Design review of the part built by this model. Coordinates are the model's own, in mm. Face numbers are marked on the shaded views. A direction names the side the tool comes from. Give positions to 0.01 mm unless a question says otherwise; leave off trailing zeros. Order: outer loops, then holes, each group sorted by start corner. A loop starts at its lowest first (then second) coordinate and runs counter-clockwise, first axis right, second up. Notation, with made-up numbers: (35, 4.25) -> (49, 4.25) arc R25 cw to (49, 37.25) -> close; hole circle Ø4 at (71.25, 22.5). An arc over 180 degrees is marked (long way). Use a Markdown table: item, result. Add a question column.
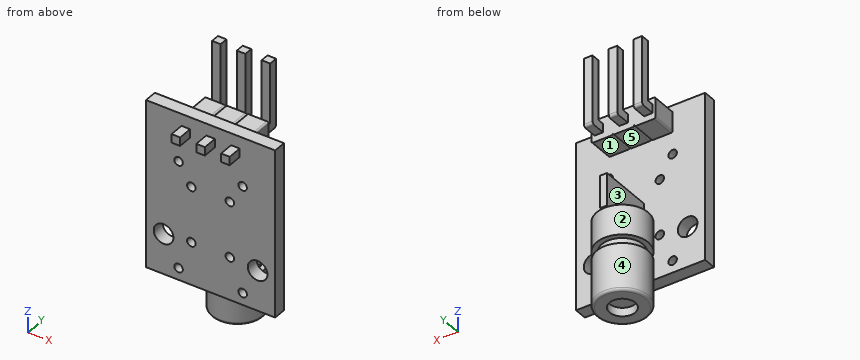
```python
from build123d import *

# Parameters (mm, degrees)
SKETCH1_W           = 15.1
SKETCH1_H           = 19.6
BOSS_EXTRUDE1_DEPTH = 1.5
SKETCH2_W           = 1
SKETCH2_H           = 1
BOSS_EXTRUDE2_DEPTH = 1.7
BOSS_EXTRUDE3_DEPTH = 2.9
SKETCH4_W           = 1
SKETCH4_H           = 1
BOSS_EXTRUDE4_DEPTH = 1.8
SKETCH5_W           = 1
SKETCH5_H           = 1
BOSS_EXTRUDE5_DEPTH = 7
SKETCH7_W           = 0.8
SKETCH7_H           = 3.8
BOSS_EXTRUDE6_DEPTH = 6.3
SKETCH8_R           = 3
BOSS_EXTRUDE7_DEPTH = 3.5
SKETCH9_R           = 2.4
BOSS_EXTRUDE8_DEPTH = 1
SKETCH10_R          = 3
BOSS_EXTRUDE9_DEPTH = 5.5
FILLET1_R           = 0.3
SKETCH11_R          = 1.5
CUT_EXTRUDE1_DEPTH  = 1
SKETCH12_R          = 1.15
CUT_EXTRUDE2_DEPTH  = 19.271631016
CUT_EXTRUDE3_REACH  = 20.842
SKETCH13_R          = 0.5
CUT_EXTRUDE4_REACH  = 20.842
SKETCH14_R          = 0.5
FILLET2_R           = 0.2
FILLET3_R           = 0.05
FILLET5_R           = 0.3


with BuildPart() as part:
    # Sketch1 → Boss-Extrude1 (new body)
    with BuildSketch(Plane(origin=(0, 0, 0), x_dir=(1, 0, 0), z_dir=(0, 1, 0))):
        Rectangle(SKETCH1_W, SKETCH1_H)
    extrude(amount=BOSS_EXTRUDE1_DEPTH)

    # Sketch2 → Boss-Extrude2 (add)
    with BuildSketch(Plane.XZ):
        with Locations((0, 7.9)):
            Rectangle(SKETCH2_W, SKETCH2_H)
        with Locations((2.9, 7.9)):
            Rectangle(SKETCH2_W, SKETCH2_H)
        with Locations((-2.9, 7.9)):
            Rectangle(SKETCH2_W, SKETCH2_H)
    extrude(amount=BOSS_EXTRUDE2_DEPTH)

    # Sketch3 → Boss-Extrude3 (add)
    with BuildSketch(Plane(origin=(0, 1.5, 0), x_dir=(1, 0, 0), z_dir=(0, 1, 0))):
        with BuildLine():
            Line((-3.75, -9.15), (-3.75, -6.65))
            Line((-3.75, -6.65), (-1.45, -6.65))
            ThreePointArc((-1.45, -6.65), (-1.308578644, -6.708578644), (-1.25, -6.85))
            ThreePointArc((-1.25, -6.85), (-1.191421356, -6.708578644), (-1.05, -6.65))
            Line((-1.05, -6.65), (1.05, -6.65))
            ThreePointArc((1.05, -6.65), (1.191421356, -6.708578644), (1.25, -6.85))
            ThreePointArc((1.25, -6.85), (1.308578644, -6.708578644), (1.45, -6.65))
            Line((1.45, -6.65), (3.75, -6.65))
            Line((3.75, -6.65), (3.75, -9.15))
            Line((3.75, -9.15), (1.45, -9.15))
            ThreePointArc((1.45, -9.15), (1.308578644, -9.091421356), (1.25, -8.95))
            ThreePointArc((1.25, -8.95), (1.191421356, -9.091421356), (1.05, -9.15))
            Line((1.05, -9.15), (-1.05, -9.15))
            ThreePointArc((-1.05, -9.15), (-1.191421356, -9.091421356), (-1.25, -8.95))
            ThreePointArc((-1.25, -8.95), (-1.308578644, -9.091421356), (-1.45, -9.15))
            Line((-1.45, -9.15), (-3.75, -9.15))
        make_face()
    extrude(amount=BOSS_EXTRUDE3_DEPTH)

    # Sketch4 → Boss-Extrude4 (add)
    with BuildSketch(Plane(origin=(0, 4.4, 0), x_dir=(1, 0, 0), z_dir=(0, 1, 0))):
        with Locations((-2.9, -7.9)):
            Rectangle(SKETCH4_W, SKETCH4_H)
        with Locations((0, -7.9)):
            Rectangle(SKETCH4_W, SKETCH4_H)
        with Locations((2.9, -7.9)):
            Rectangle(SKETCH4_W, SKETCH4_H)
    extrude(amount=BOSS_EXTRUDE4_DEPTH)

    # Sketch5 → Boss-Extrude5 (add)
    with BuildSketch(Plane.XY.offset(8.4)):
        with Locations((-2.9, 5.7)):
            Rectangle(SKETCH5_W, SKETCH5_H)
        with Locations((0, 5.7)):
            Rectangle(SKETCH5_W, SKETCH5_H)
        with Locations((2.9, 5.7)):
            Rectangle(SKETCH5_W, SKETCH5_H)
    extrude(amount=BOSS_EXTRUDE5_DEPTH)

    # Sketch7 → Boss-Extrude6 (add)
    with BuildSketch(Plane(origin=(0, 1.5, 0), x_dir=(1, 0, 0), z_dir=(0, 1, 0))):
        with Locations((0, 2.3)):
            Rectangle(SKETCH7_W, SKETCH7_H)
    extrude(amount=BOSS_EXTRUDE6_DEPTH)

    # Sketch8 → Boss-Extrude7 (add)
    with BuildSketch(Plane(origin=(0, 0, -4.2), x_dir=(-1, 0, 0), z_dir=(0, 0, -1))):
        with Locations(Location((0, 4.6, 0), (0, 0, 262.337744339))):
            Circle(SKETCH8_R)
    extrude(amount=BOSS_EXTRUDE7_DEPTH)

    # Sketch9 → Boss-Extrude8 (add)
    with BuildSketch(Plane(origin=(0, 0, -7.7), x_dir=(-1, 0, 0), z_dir=(0, 0, -1))):
        with Locations((0, 4.6)):
            Circle(SKETCH9_R)
    extrude(amount=BOSS_EXTRUDE8_DEPTH)

    # Sketch10 → Boss-Extrude9 (add)
    with BuildSketch(Plane(origin=(0, 0, -8.7), x_dir=(-1, 0, 0), z_dir=(0, 0, -1))):
        with Locations(Location((0, 4.6, 0), (0, 0, 262.337744339))):
            Circle(SKETCH10_R)
    extrude(amount=BOSS_EXTRUDE9_DEPTH)

    # Fillet1
    fillet1_edges = [part.edges().sort_by_distance(p)[0] for p in [
        (-0.4, 7.573213749, -14.2),
    ]]
    fillet(fillet1_edges, radius=FILLET1_R)

    # Sketch11 → Cut-Extrude1 (cut)
    with BuildSketch(Plane(origin=(0, 0, -14.2), x_dir=(-1, 0, 0), z_dir=(0, 0, -1))):
        with Locations((0, 4.6)):
            Circle(SKETCH11_R)
    extrude(amount=-CUT_EXTRUDE1_DEPTH, mode=Mode.SUBTRACT)

    # Sketch12 → Cut-Extrude2 (cut, through all)
    with BuildSketch(Plane(origin=(0, 1.5, 0), x_dir=(1, 0, 0), z_dir=(0, 1, 0))):
        with Locations(Location((-5.5, 5.1, 0), (0, 0, 270))):
            Circle(SKETCH12_R)
        with Locations(Location((5.5, 5.1, 0), (0, 0, 270))):
            Circle(SKETCH12_R)
    extrude(amount=-CUT_EXTRUDE2_DEPTH, mode=Mode.SUBTRACT)

    # Sketch13 → Cut-Extrude3 (cut, up to next)
    with BuildSketch(Plane.XZ, mode=Mode.PRIVATE) as cut_extrude3_sk1:
        with Locations(Location((-2.25, -4.8, 0), (0, 0, 270))):
            Circle(SKETCH13_R)
    cut_extrude3_tool1 = extrude(cut_extrude3_sk1.sketch, amount=-CUT_EXTRUDE3_REACH, mode=Mode.PRIVATE) & part.part
    # Sketch13 → Cut-Extrude3 (cut, up to next)
    with BuildSketch(Plane.XZ, mode=Mode.PRIVATE) as cut_extrude3_sk2:
        with Locations(Location((2.25, -4.8, 0), (0, 0, 270))):
            Circle(SKETCH13_R)
    cut_extrude3_tool2 = extrude(cut_extrude3_sk2.sketch, amount=-CUT_EXTRUDE3_REACH, mode=Mode.PRIVATE) & part.part
    # Sketch13 → Cut-Extrude3 (cut, up to next)
    with BuildSketch(Plane.XZ, mode=Mode.PRIVATE) as cut_extrude3_sk3:
        with Locations(Location((2.25, 1.7, 0), (0, 0, 270))):
            Circle(SKETCH13_R)
    cut_extrude3_tool3 = extrude(cut_extrude3_sk3.sketch, amount=-CUT_EXTRUDE3_REACH, mode=Mode.PRIVATE) & part.part
    # Sketch13 → Cut-Extrude3 (cut, up to next)
    with BuildSketch(Plane.XZ, mode=Mode.PRIVATE) as cut_extrude3_sk4:
        with Locations(Location((-2.25, 1.7, 0), (0, 0, 270))):
            Circle(SKETCH13_R)
    cut_extrude3_tool4 = extrude(cut_extrude3_sk4.sketch, amount=-CUT_EXTRUDE3_REACH, mode=Mode.PRIVATE) & part.part
    add(cut_extrude3_tool1.solids().sort_by_distance((-2.25, 0, -4.8))[0], mode=Mode.SUBTRACT)
    add(cut_extrude3_tool2.solids().sort_by_distance((2.25, 0, -4.8))[0], mode=Mode.SUBTRACT)
    add(cut_extrude3_tool3.solids().sort_by_distance((2.25, 0, 1.7))[0], mode=Mode.SUBTRACT)
    add(cut_extrude3_tool4.solids().sort_by_distance((-2.25, 0, 1.7))[0], mode=Mode.SUBTRACT)

    # Sketch14 → Cut-Extrude4 (cut, up to next)
    with BuildSketch(Plane.XZ, mode=Mode.PRIVATE) as cut_extrude4_sk1:
        with Locations(Location((3.75, 4.1, 0), (0, 0, 270))):
            Circle(SKETCH14_R)
    cut_extrude4_tool1 = extrude(cut_extrude4_sk1.sketch, amount=-CUT_EXTRUDE4_REACH, mode=Mode.PRIVATE) & part.part
    # Sketch14 → Cut-Extrude4 (cut, up to next)
    with BuildSketch(Plane.XZ, mode=Mode.PRIVATE) as cut_extrude4_sk2:
        with Locations(Location((-3.75, 4.1, 0), (0, 0, 270))):
            Circle(SKETCH14_R)
    cut_extrude4_tool2 = extrude(cut_extrude4_sk2.sketch, amount=-CUT_EXTRUDE4_REACH, mode=Mode.PRIVATE) & part.part
    # Sketch14 → Cut-Extrude4 (cut, up to next)
    with BuildSketch(Plane.XZ, mode=Mode.PRIVATE) as cut_extrude4_sk3:
        with Locations(Location((-3.75, -8.4, 0), (0, 0, 270))):
            Circle(SKETCH14_R)
    cut_extrude4_tool3 = extrude(cut_extrude4_sk3.sketch, amount=-CUT_EXTRUDE4_REACH, mode=Mode.PRIVATE) & part.part
    # Sketch14 → Cut-Extrude4 (cut, up to next)
    with BuildSketch(Plane.XZ, mode=Mode.PRIVATE) as cut_extrude4_sk4:
        with Locations(Location((3.75, -8.4, 0), (0, 0, 270))):
            Circle(SKETCH14_R)
    cut_extrude4_tool4 = extrude(cut_extrude4_sk4.sketch, amount=-CUT_EXTRUDE4_REACH, mode=Mode.PRIVATE) & part.part
    add(cut_extrude4_tool1.solids().sort_by_distance((3.75, 0, 4.1))[0], mode=Mode.SUBTRACT)
    add(cut_extrude4_tool2.solids().sort_by_distance((-3.75, 0, 4.1))[0], mode=Mode.SUBTRACT)
    add(cut_extrude4_tool3.solids().sort_by_distance((-3.75, 0, -8.4))[0], mode=Mode.SUBTRACT)
    add(cut_extrude4_tool4.solids().sort_by_distance((3.75, 0, -8.4))[0], mode=Mode.SUBTRACT)

    # Fillet2
    fillet2_edges = [part.edges().sort_by_distance(p)[0] for p in [
        (-3.75, 2.95, 9.15),
        (3.75, 2.95, 9.15),
        (3.75, 2.95, 6.65),
        (-3.75, 2.95, 6.65),
    ]]
    fillet(fillet2_edges, radius=FILLET2_R)

    # Fillet3
    fillet3_edges = [part.edges().sort_by_distance(p)[0] for p in [
        (-2.9, 5.2, 8.4),
        (0, 5.2, 8.4),
        (2.9, 5.2, 8.4),
    ]]
    fillet(fillet3_edges, radius=FILLET3_R)

    # Fillet5
    fillet5_edges = [part.edges().sort_by_distance(p)[0] for p in [
        (-2.9, 6.2, 7.4),
        (0, 6.2, 7.4),
        (2.9, 6.2, 7.4),
    ]]
    fillet(fillet5_edges, radius=FILLET5_R)


solid = part.part
```
1) Add section B-B (z = 4.1). Give the boundary of the cut face in (x, y).
2) Add section D-D (z = -4.8). Give the boundary of the cut face in (x, y).
3) The part is to be moulded in two halves that separate along Z. For the marked faces 4 and 5, say which applies: +Z half, -Z half, draft (parallel to the pull), parting line (faces both ways), or undercut.
4) Machinability: for the marked faces 1, 2 and 3, which of the approach directions +Z, -Z, +X, -X, +Y, -Y give a long, thin tool a straight path to every point of the face, cutting with its end or side? Answer none if there is none.
5) Add section A-A (y = 1). Give the number of separate pieces and of enclosed holes in the cut face, then the cut area to 3 significant figures.
6) Insertion check: pin 1 (1 mm diameter, centred on x = 2, y = 2.5, fed in from +Z); pin 2 (4 mm diameter, centred on y = 7, z = -4, fed in from -X); pin 3 (0.5 mm diameter, centred on y = 5.5, z = 10.5, fed in from +X); pin 4 (5 mm diameter, centred on y = 2.5, z = -9.5, fed in from +X). Each pin has a flat end and moves straight along its axis. Give the tip position at first contact, or say it passes through.
7) For L1, parallel to Y at x = 0, z = -13.35; L2, parallel to X at y = 0.5, z = -5.75; L3, parallel to Z at x = 0.25, y = 5, list the stretches that pass through material, from the lowest coordinate up. Write a range as [from, to].
8) Add section C-C (y = -1). Give the boundary of the cut face in (x, z), then the cut area to 3 significant figures.
Worked answers:
| question | item | result |
|---|---|---|
| 1 | outline | (-7.55, 0) -> (-4.25, 0) -> (-4.25, 1.5) -> (-7.55, 1.5) -> close; (-3.25, 0) -> (3.25, 0) -> (3.25, 1.5) -> (-3.25, 1.5) -> close; (4.25, 0) -> (7.55, 0) -> (7.55, 1.5) -> (4.25, 1.5) -> close |
| 2 | outline | (-7.55, 0) -> (-6.61, 0) -> (-6.61, 1.5) -> (-7.55, 1.5) -> close; (-4.39, 0) -> (-2.75, 0) -> (-2.75, 1.5) -> (-4.39, 1.5) -> close; circle Ø6 at (0, 4.6); (-1.75, 0) -> (1.75, 0) -> (1.75, 1.5) -> (-1.75, 1.5) -> close; (2.75, 0) -> (4.39, 0) -> (4.39, 1.5) -> (2.75, 1.5) -> close; (6.61, 0) -> (7.55, 0) -> (7.55, 1.5) -> (6.61, 1.5) -> close |
| 3 | face 4 | draft |
| 3 | face 5 | undercut |
| 4 | face 1 | +X, -X, +Y |
| 4 | face 2 | -Z |
| 4 | face 3 | -X, +Y |
| 5 | separate pieces | 1 |
| 5 | enclosed holes | 10 |
| 5 | area | 281 mm^2 |
| 6 | pin 1 | z = 9.15 |
| 6 | pin 2 | x = -2.97 |
| 6 | pin 3 | x = 3.4 |
| 6 | pin 4 | x = 7.55 |
| 7 | L1 | [1.6, 3.1], [6.1, 7.6] |
| 7 | L2 | [-7.55, -6.45], [-4.55, 4.55], [6.45, 7.55] |
| 7 | L3 | [-13.2, -0.4], [7.4, 8.4] |
| 8 | outline | (-3.4, 7.4) -> (-2.4, 7.4) -> (-2.4, 8.4) -> (-3.4, 8.4) -> close; (-0.5, 7.4) -> (0.5, 7.4) -> (0.5, 8.4) -> (-0.5, 8.4) -> close; (2.4, 7.4) -> (3.4, 7.4) -> (3.4, 8.4) -> (2.4, 8.4) -> close |
| 8 | area | 3.00 mm^2 |
